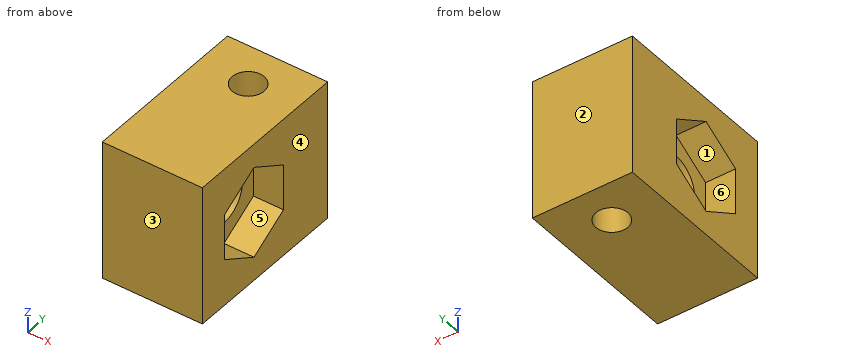
from build123d import *

# Parameters (mm, degrees)
SKETCH1_W           = 10
SKETCH1_H           = 17
BOSS_EXTRUDE1_DEPTH = 14
SKETCH2_R           = 1.6
CUT_EXTRUDE1_DEPTH  = 15
CUT_EXTRUDE2_DEPTH  = 3
SKETCH5_R           = 2.5
CUT_EXTRUDE3_DEPTH  = 8


with BuildPart() as part:
    # Sketch1 → Boss-Extrude1 (new body)
    with BuildSketch(Plane.XY):
        Rectangle(SKETCH1_W, SKETCH1_H)
    extrude(amount=BOSS_EXTRUDE1_DEPTH)

    # Sketch2 → Cut-Extrude1 (cut, through all)
    with BuildSketch(Plane(origin=(0, 0, 0), x_dir=(-1, 0, 0), z_dir=(0, 0, -1))):
        with Locations((0, 4.5)):
            Circle(SKETCH2_R)
    extrude(amount=-CUT_EXTRUDE1_DEPTH, mode=Mode.SUBTRACT)

    # Sketch3 → Cut-Extrude2 (cut)
    with BuildSketch(Plane.ZY.offset(5)):
        Polygon((2.381197846, -1.5), (4.690598923, -5.5), (9.309401077, -5.5), (11.618802154, -1.5), (9.309401077, 2.5), (4.690598923, 2.5), align=None)
    cut_extrude2 = extrude(amount=-CUT_EXTRUDE2_DEPTH, mode=Mode.SUBTRACT)

    # Sketch5 → Cut-Extrude3 (cut, through all)
    with BuildSketch(Plane.ZY.offset(2)):
        with Locations((7, -1.5)):
            Circle(SKETCH5_R)
    extrude(amount=-CUT_EXTRUDE3_DEPTH, mode=Mode.SUBTRACT)

    # Mirror1: Cut-Extrude2 across plane
    add(cut_extrude2.mirror(Plane(origin=(0, 0, 0), x_dir=(0, 0, 1), z_dir=(1, 0, 0))), mode=Mode.SUBTRACT)


solid = part.part
Here's how the part is built. I have some questions about the finished solid (model axes, mm). Face numbers are marked on the shaded views. A direction names the side the tool comes from. Coordinates: 2 decimals unless noted, no trailing zeros. Write each loop counter-clockwise with the first axis right and the second up, starting at its lowest first coordinate (ties: lowest second). Pieces come first, ordered by that corner, then holes.
1) Which directions (+Z, -Z, +X, -X, +Y, -Y) give clear straight access to the entire face, cutting with the end or side of a thin tool? Please do the marked faces 4, 5 and 6.
Filled in:
face 4: +Z, -Z, +X, +Y, -Y
face 5: +X
face 6: -X
2) If I drill on line 1 (Y direction, x = 0.35, z = 7); line 2 (Y direction, x = 0, z = 6.25); line 3 (X direction, y = -2, z = 10.5), over which ranges is the centre line in solid material (lowest first)?
Filled in:
line 1: y = -8.5 to -4, 1 to 2.94, 6.06 to 8.5
line 2: y = -8.5 to -3.88, 0.88 to 2.9, 6.1 to 8.5
line 3: x = -2 to 2
3) If we section it at C-C (y = 4.5): List the corners of the cut face in (x, z) for me, plus the area to 3 significant figures.
Filled in:
outline: (-5, 0) - (-1.6, 0) - (-1.6, 14) - (-5, 14) - close; (1.6, 0) - (5, 0) - (5, 14) - (1.6, 14) - close
area: 95.2 mm2
4) Thinking about a two-plate mould opening in Y: for the marked faces 1, 2 and 3, which applies, +Y half, -Y half, draft (parallel to the pull), parting line (faces both ways), or undercut?
Filled in:
face 1: undercut
face 2: +Y half
face 3: -Y half
5) If we section it at B-B (z = 8.5): List the corners of the cut face in (x, y) for me, plus the area to 3 significant figures.
Filled in:
outline: (-5, -8.5) - (5, -8.5) - (5, -5.5) - (2, -5.5) - (2, -3.5) - (-2, -3.5) - (-2, -5.5) - (-5, -5.5) - close; (-5, 2.5) - (-2, 2.5) - (-2, 0.5) - (2, 0.5) - (2, 2.5) - (5, 2.5) - (5, 8.5) - (-5, 8.5) - close; hole circle Ø3.2 at (0, 4.5)
area: 98.0 mm2
6) If we section it at D-D (x = -2.75): List the corners of the cut face in (y, z) for me, plus the area to 3 significant figures.
Filled in:
outline: (-8.5, 0) - (8.5, 0) - (8.5, 14) - (-8.5, 14) - close; hole (-5.5, 4.69) - (-1.5, 2.38) - (2.5, 4.69) - (2.5, 9.31) - (-1.5, 11.62) - (-5.5, 9.31) - close
area: 183 mm2
7) If we section it at A-A (x = 0): List the corners of the cut face in (y, z) for me.
Filled in:
outline: (-8.5, 0) - (2.9, 0) - (2.9, 14) - (-8.5, 14) - close; (6.1, 0) - (8.5, 0) - (8.5, 14) - (6.1, 14) - close; hole circle Ø5 at (-1.5, 7)
8) I'm going to push flat-ended pins straight in: pin 1 (3 mm diameter, centred on x = 0, y = 4.5, fed in from -Z); pin 2 (1.5 mm diameter, centred on y = -0.5, z = 5.5, fed in from +X); pin 3 (4 mm diameter, centred on y = -0.5, z = 6, fed in from -X). Where does each tip first touch, or does it pass through?
Filled in:
pin 1: passes through
pin 2: stops at x = 2
pin 3: stops at x = -2
